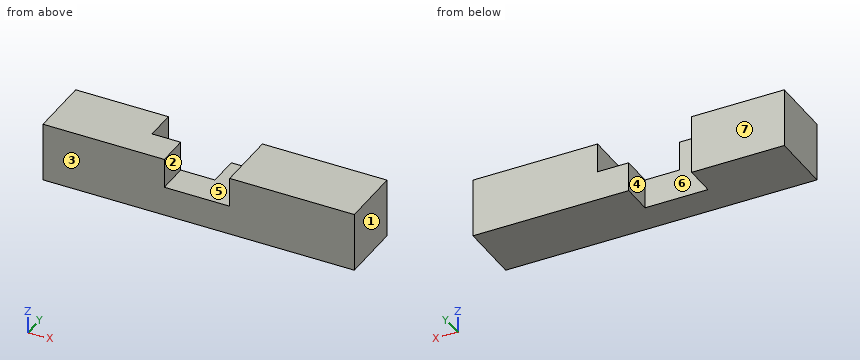
from build123d import *

# Parameters (mm, degrees)
SKETCH_1_W           = 100
SKETCH_1_H           = 20
EXTRUDE_1_DEPTH      = 19
SKETCH_2_W           = 30
SKETCH_2_H           = 9
CUT_EXTRUDE_8_DEPTH  = 36.5
SKETCH_7_W           = 11
SKETCH_7_H           = 19
CUT_EXTRUDE_9_DEPTH  = 10
SKETCH_8_W           = 20
SKETCH_8_H           = 10
CUT_EXTRUDE_10_DEPTH = 10
SKETCH_9_W           = 11
SKETCH_9_H           = 19
EXTRUDE_3_DEPTH      = 10
SKETCH_10_W          = 10
SKETCH_10_H          = 10
EXTRUDE_4_DEPTH      = 10
SKETCH_11_W          = 10
SKETCH_11_H          = 10
CUT_EXTRUDE_11_DEPTH = 10
SKETCH_16_W          = 9
SKETCH_16_H          = 20
EXTRUDE_8_DEPTH      = 10
SKETCH_17_W          = 10
SKETCH_17_H          = 10
EXTRUDE_9_DEPTH      = 20
SKETCH_12_W          = 10
SKETCH_12_H          = 9
CUT_EXTRUDE_12_DEPTH = 21
SKETCH_19_W          = 10.2
SKETCH_19_H          = 19
CUT_EXTRUDE_16_DEPTH = 10
SKETCH_20_W          = 9
SKETCH_20_H          = 20
EXTRUDE_10_DEPTH     = 10
SKETCH_21_W          = 11
SKETCH_21_H          = 10.5
CUT_EXTRUDE_17_DEPTH = 10
SKETCH_22_W          = 0.5
SKETCH_22_H          = 20
CUT_EXTRUDE_18_DEPTH = 10
SHELL_1_T            = -2
SKETCH_23_W          = 15
SKETCH_23_H          = 16
EXTRUDE_11_DEPTH     = 2


with BuildPart() as part:
    # 草圖1 → 填料-伸長1 (new body)
    with BuildSketch(Plane.XY):
        Rectangle(SKETCH_1_W, SKETCH_1_H)
    extrude(amount=EXTRUDE_1_DEPTH)

    # 草圖2 → 除料-伸長8 (cut)
    with BuildSketch(Plane(origin=(0, 10, 0), x_dir=(1, 0, 0), z_dir=(0, 1, 0))):
        with Locations((4.974315736, -14.5)):
            Rectangle(SKETCH_2_W, SKETCH_2_H)
    extrude(amount=-CUT_EXTRUDE_8_DEPTH, mode=Mode.SUBTRACT)

    # 草圖7 → 除料-伸長9 (cut)
    with BuildSketch(Plane(origin=(0, 10, 0), x_dir=(1, 0, 0), z_dir=(0, 1, 0))):
        with Locations((-15.525684264, -9.5)):
            Rectangle(SKETCH_7_W, SKETCH_7_H)
    extrude(amount=-CUT_EXTRUDE_9_DEPTH, mode=Mode.SUBTRACT)

    # 草圖8 → 除料-伸長10 (cut)
    with BuildSketch(Plane(origin=(0, 10, 0), x_dir=(1, 0, 0), z_dir=(0, 1, 0))):
        with Locations((-0.025684264, -5)):
            Rectangle(SKETCH_8_W, SKETCH_8_H)
    extrude(amount=-CUT_EXTRUDE_10_DEPTH, mode=Mode.SUBTRACT)

    # 草圖9 → 填料-伸長3 (add)
    with BuildSketch(Plane(origin=(0, 0, 0), x_dir=(1, 0, 0), z_dir=(0, 1, 0))):
        with Locations((-15.525684264, -9.5)):
            Rectangle(SKETCH_9_W, SKETCH_9_H)
    extrude(amount=EXTRUDE_3_DEPTH)

    # 草圖10 → 填料-伸長4 (add)
    with BuildSketch(Plane(origin=(-10.025684264, 0, 0), x_dir=(0, 0, -1), z_dir=(1, 0, 0))):
        with Locations((-15, -5)):
            Rectangle(SKETCH_10_W, SKETCH_10_H)
    extrude(amount=EXTRUDE_4_DEPTH)

    # 草圖11 → 除料-伸長11 (cut)
    with BuildSketch(Plane(origin=(0, 10, 0), x_dir=(1, 0, 0), z_dir=(0, 1, 0))):
        with Locations((14.974315736, -5)):
            Rectangle(SKETCH_11_W, SKETCH_11_H)
    extrude(amount=-CUT_EXTRUDE_11_DEPTH, mode=Mode.SUBTRACT)

    # 草圖16 → 填料-伸長8 (add)
    with BuildSketch(Plane.ZY.offset(-19.974315736)):
        with Locations((14.5, 0)):
            Rectangle(SKETCH_16_W, SKETCH_16_H)
    extrude(amount=EXTRUDE_8_DEPTH)

    # 草圖17 → 填料-伸長9 (add)
    with BuildSketch(Plane.ZY.offset(-19.974315736)):
        with Locations((5, 5)):
            Rectangle(SKETCH_17_W, SKETCH_17_H)
    extrude(amount=EXTRUDE_9_DEPTH)

    # 草圖12 → 除料-伸長12 (cut)
    with BuildSketch(Plane(origin=(0, 10, 0), x_dir=(1, 0, 0), z_dir=(0, 1, 0))):
        with Locations((24.974315736, -14.5)):
            Rectangle(SKETCH_12_W, SKETCH_12_H)
    extrude(amount=-CUT_EXTRUDE_12_DEPTH, mode=Mode.SUBTRACT)

    # 草圖19 → 除料-伸長16 (cut)
    with BuildSketch(Plane(origin=(0, 10, 0), x_dir=(1, 0, 0), z_dir=(0, 1, 0))):
        with Locations((-15.125684264, -9.5)):
            Rectangle(SKETCH_19_W, SKETCH_19_H)
    extrude(amount=-CUT_EXTRUDE_16_DEPTH, mode=Mode.SUBTRACT)

    # 草圖20 → 填料-伸長10 (add)
    with BuildSketch(Plane.ZY.offset(-29.974315736)):
        with Locations((14.5, 0)):
            Rectangle(SKETCH_20_W, SKETCH_20_H)
    extrude(amount=EXTRUDE_10_DEPTH)

    # 草圖21 → 除料-伸長17 (cut)
    with BuildSketch(Plane(origin=(0, 0, 0), x_dir=(1, 0, 0), z_dir=(0, 1, 0))):
        with Locations((-5.525684264, -14.75)):
            Rectangle(SKETCH_21_W, SKETCH_21_H)
    extrude(amount=-CUT_EXTRUDE_17_DEPTH, mode=Mode.SUBTRACT)

    # 草圖22 → 除料-伸長18 (cut)
    with BuildSketch(Plane.ZY.offset(0.025684264)):
        with Locations((9.75, 0)):
            Rectangle(SKETCH_22_W, SKETCH_22_H)
    extrude(amount=-CUT_EXTRUDE_18_DEPTH, mode=Mode.SUBTRACT)

    # 薄殼1
    shell_1_openings = [part.faces().sort_by_distance(p)[0] for p in [
        (50, 0, 9.5),
    ]]
    offset(amount=SHELL_1_T, openings=shell_1_openings, kind=Kind.INTERSECTION)

    # 草圖23 → 填料-伸長11 (add)
    with BuildSketch(Plane(origin=(50, 0, 0), x_dir=(0, 0, -1), z_dir=(1, 0, 0))):
        with Locations((-9.5, 0)):
            Rectangle(SKETCH_23_W, SKETCH_23_H)
    extrude(amount=-EXTRUDE_11_DEPTH)


solid = part.part
Input: part model. Units: mm. Frame: model coordinates. Face numbers are marked on the shaded views. A direction names the side the tool comes from. Coordinates: 2 decimals unless noted, no trailing zeros. Loops run counter-clockwise (first coordinate to the right, second up) from the corner with the lowest first, then second, coordinate; pieces in that order, holes last. Notation, with made-up numbers: (46.25, 35) - (102.25, 35) arc R27 ccw to (102.25, 68) - close; hole circle Ø4 at (-38.5, 66). An arc over 180 degrees is marked (long way). Answer in a Markdown table with one row per item. Add a question column.
Item 1: Section query B-B on z = 12. Return the cut outline in (x, y).
Item 2: Section query D-D on y = -4. Return the cut outline in (x, z).
Item 3: Line query: line 1 along X through (y, z) = (-4.5, 14.5); line 2 along X through (y, z) = (7, 7); line 3 along X through (y, z) = (-1.75, 8). Output: solid intervals per line, ascending. Write a range as [from, to].
Item 4: Section query C-C on x = 31. Return the cut outline in (y, z), then the cut area to 3 significant figures.
Item 5: Mould query, pull axis X, two halves, no side actions, for the marked faces 1, 2, 3 and 4. Classes: released by +X, released by -X, zero draft, split by the parting line, or undercut.
Item 6: Access query for the marked faces 5, 6 and 7. Directions: +Z, -Z, +X, -X, +Y, -Y. A direction counts if a zero-diameter tool reaches every point of the face in a straight line with its end or side. Return the directions, or none.
Item 7: Section query A-A on y = 4.5. Return the cut outline in (x, z).
Item 8: Contact query for flat-ended pins moving along their axis: P1, Ø4.5, axis at x = -12.5, z = 6, coming from the +Y side; P2, Ø6, axis at x = -4.5, y = -1.5, coming from the +Z side. Output: stop coordinate, or through.
Recorded:
| question | item | result |
|---|---|---|
| 1 | outline | (-50, -10) - (-11.03, -10) - (-11.03, 0) - (-20.23, 0) - (-20.23, 10) - (-50, 10) - close; (9.97, -10) - (50, -10) - (50, 10) - (9.97, 10) - close; hole (-48, -8) - (-13.03, -8) - (-13.03, -2) - (-22.23, -2) - (-22.23, 8) - (-48, 8) - close; hole (11.97, -8) - (48, -8) - (48, 8) - (11.97, 8) - close |
| 2 | outline | (-50, 0) - (50, 0) - (50, 19) - (9.97, 19) - (9.97, 9.5) - (-11.03, 9.5) - (-11.03, 19) - (-50, 19) - close; hole (-48, 2) - (48, 2) - (48, 17) - (11.97, 17) - (11.97, 7.5) - (-13.03, 7.5) - (-13.03, 17) - (-48, 17) - close |
| 3 | line 1 | [-50, -48], [-13.03, -11.03], [9.97, 11.97], [48, 50] |
| 3 | line 2 | [-50, -48], [-22.23, -20.23], [-0.03, 1.97], [48, 50] |
| 3 | line 3 | [-50, -48], [-22.23, 11.97], [48, 50] |
| 4 | outline | (-10, 0) - (10, 0) - (10, 19) - (-10, 19) - close; hole (-8, 2) - (8, 2) - (8, 17) - (-8, 17) - close |
| 4 | area | 140 mm^2 |
| 5 | face 1 | released by +X |
| 5 | face 2 | undercut |
| 5 | face 3 | zero draft |
| 5 | face 4 | undercut |
| 6 | face 5 | +Z, +Y, -Y |
| 6 | face 6 | +Z, -Z, +Y |
| 6 | face 7 | +Z, -Z, +X, -X, +Y |
| 7 | outline | (-50, 0) - (-20.23, 0) - (-20.23, 19) - (-50, 19) - close; (-0.03, 0) - (50, 0) - (50, 19) - (9.97, 19) - (9.97, 9.5) - (-0.03, 9.5) - close; hole (-48, 2) - (-22.23, 2) - (-22.23, 17) - (-48, 17) - close; hole (1.97, 2) - (48, 2) - (48, 17) - (11.97, 17) - (11.97, 7.5) - (1.97, 7.5) - close |
| 8 | P1 | y = 0 |
| 8 | P2 | z = 9.5 |
